from build123d import *

# Parameters (mm, degrees)
F1_DEPTH = 19
F3_DEPTH = 9


with BuildPart() as f1:
    # F0 (on Front) → F1 (new body)
    with BuildSketch(Plane.XZ):
        with BuildLine():
            Line((215.803112, -98.339818), (215.803112, 91.660182))
            Line((215.803112, 91.660182), (40.803112, 91.660182))
            ThreePointArc((40.803112, 91.660182), (-51.188735, 51.467448), (-84.196888, -43.339818))
            Line((-84.196888, -43.339818), (-84.196888, -98.339818))
            Line((-84.196888, -98.339818), (215.803112, -98.339818))
        make_face()
    extrude(amount=F1_DEPTH)

    # F2 (on face) → F3 (cut)
    with BuildSketch(Plane.XZ.offset(19)):
        with BuildLine():
            Line((-48.476428, -98.339818), (-48.476428, -43.339818))
            ThreePointArc((-48.476428, -43.339818), (-23.380529, 27.820504), (40.803112, 67.494877))
            Line((40.803112, 67.494877), (215.803112, 67.494877))
            Line((215.803112, 67.494877), (215.803112, 83.558917))
            Line((215.803112, 83.558917), (40.803112, 83.558917))
            ThreePointArc((40.803112, 83.558917), (-37.824855, 40.607519), (-69.130197, -43.339818))
            Line((-69.130197, -43.339818), (-69.130197, -98.339818))
            Line((-69.130197, -98.339818), (-48.476428, -98.339818))
        make_face()
    extrude(amount=-F3_DEPTH, mode=Mode.SUBTRACT)


solid = f1.part
Part model, mm, in its own coordinate system. A direction names the side the tool comes from. Coordinates: 2 decimals unless noted, no trailing zeros. Order: outer loops, then holes, each group sorted by start corner. A loop starts at its lowest first (then second) coordinate and runs counter-clockwise, first axis right, second up. Notation, with made-up numbers: M 0,87 L 5,87 A20 cw 5,92 Z; hole C 83,0.5 d11. An arc over 180 degrees is marked long. One line per question, with ' | ' between items.
Q1. Slice it at A-A (y = -14.5). Give the cut face in (x, z), and give its area (3 significant figures).
A:
outline: M -84.2,-98.34 L -69.13,-98.34 L -69.13,-43.34 A128.21 cw 40.8,83.56 L 215.8,83.56 L 215.8,91.66 L 40.8,91.66 A125.37 ccw -84.2,-43.34 Z; M -48.48,-98.34 L 215.8,-98.34 L 215.8,67.49 L 40.8,67.49 A113.44 ccw -48.48,-43.34 Z | area: 46,500 mm^2
Q2. Drill centre lines: line 1 (Z direction, x = 157, y = -15); line 2 (Z direction, x = 40.5, y = -16.5); line 3 (X direction, y = -12.75, z = -56.5). Where is each one in solid material? Low to high.
A:
line 1: z = -98.34 to 67.49, 83.56 to 91.66 | line 2: z = -98.34 to 67.43, 83.51 to 91.66 | line 3: x = -84.2 to -69.13, -48.48 to 215.8
Q3. Slice it at C-C (z = -80.5). Give the cut face in (x, y).
A:
outline: M -84.2,-19 L -69.13,-19 L -69.13,-10 L -48.48,-10 L -48.48,-19 L 215.8,-19 L 215.8,0 L -84.2,0 Z
Q4. Two-plate mould, pull along Z, no slides. Class faces 6 (the face through (64, -9, -98.34)), 7 (the face through (130, -15, 83.559)), 8 (the face through (-69.13, -15, -70)): +Z half, -Z half, draft (parallel to the pull), parting line (faces both ways), or undercut.
A:
face 6: -Z half | face 7: undercut | face 8: draft
Q5. Slice it at B-B (x = 114). Give the cut face in (y, z).
A:
outline: M -19,-98.34 L 0,-98.34 L 0,91.66 L -19,91.66 L -19,83.56 L -10,83.56 L -10,67.49 L -19,67.49 Z
Q6. Pin check, flat tips, straight feed: P1, Ø6, axis at y = -15.5, z = -3.5, coming from the -X side; P2, Ø10, axis at y = -16.5, z = -84, coming from the -X side. Stop position of each tip, or through.
A:
P1: stops at x = -81.58 | P2: stops at x = -84.2
Q7. 3-axis set-ups, long thin cutter, end or side, ignore diameter. For faces 1 (the face through (-48.476, -15, -71)), 2 (the face through (127, -15, 67.495)), 3 (the face through (130, -9, 91.66)), 4 (the face through (-84.197, -9, -70)), 5 (the face through (-24.05, -14.56, 26.98)): which of +Z, -Z, +X, -X, +Y, -Y reach the whole face in a straight line?
A:
face 1: -Z, -Y | face 2: +X, -Y | face 3: +Z, +X, -X, +Y, -Y | face 4: -Z, -X, +Y, -Y | face 5: -Y
